Model file for the job. Use its own axes, mm. A direction names the side the tool comes from. Give positions to 0.01 mm unless a question says otherwise; leave off trailing zeros. Write each loop counter-clockwise with the first axis right and the second up, starting at its lowest first coordinate (ties: lowest second). Pieces come first, ordered by that corner, then holes.
```python
from build123d import *

# Parameters (mm, degrees)
F2_R      = 0.3
F3_DEPTH  = 2
F4_DEPTH  = 25
F5_R      = 0.3
F6_ANGLE  = 90
F6_FACE_R = 0.3
F7_R      = 0.3
F8_DEPTH  = 3


# Not quite as in the source:
# - a feature names something its author has since deleted; it is built from what else it names


with BuildPart() as f1:
    # F0 (on Front) → F1 (revolve)
    with BuildSketch(Plane.XZ):
        with BuildLine():
            Line((0, 3.6), (0, 0))
            Line((0, 0), (1.5, 0))
            Line((1.5, 0), (2, 0))
            Line((2, 0), (2, 1))
            Line((2, 1), (1.5, 1))
            Line((1.5, 1), (1.5, 3.6))
            ThreePointArc((1.5, 3.6), (1.0606601718, 4.6606601718), (0, 5.1))
            Line((0, 5.1), (0, 3.6))
        make_face()
    revolve(axis=Axis((0, 0, 1.8), (0, 0, 1)))

    # F2 (on Top) → F3 (join)
    with BuildSketch(Plane.XY):
        with Locations((-1.27, 0)):
            Circle(F2_R)
        with Locations((1.27, 0)):
            Circle(F2_R)
    extrude(amount=-F3_DEPTH)

    # F2 (on Top) → F4 (cut)
    with BuildSketch(Plane.XY):
        with BuildLine():
            Line((1.65, 1.1302654555), (1.65, 0))
            Line((1.65, 0), (1.65, -1.1302654555))
            ThreePointArc((1.65, -1.1302654555), (1.9104973175, -0.5916079783), (2, 0))
            ThreePointArc((2, 0), (1.9104973175, 0.5916079783), (1.65, 1.1302654555))
        make_face()
    extrude(amount=F4_DEPTH, mode=Mode.SUBTRACT)

    # F5 (on face) → F6 (revolve)
    with BuildSketch(Plane(origin=(0, 0, -2), x_dir=(1, 0, 0), z_dir=(0, 0, -1))):
        with Locations((-1.27, 0)):
            Circle(F5_R)
        with Locations((1.27, 0)):
            Circle(F5_R)
    revolve(axis=Axis((0.0564431539, 1.5424509184, -2), (1, 0, 0)), revolution_arc=F6_ANGLE)

    # F6_face (on face) + F7 (on face) → F8 (join)
    with BuildSketch(Plane(origin=(1.27, 1.5424509184, -3.5424509184), x_dir=(-1, 0, 0), z_dir=(0, 1, 0))):
        with Locations((2.54, 0)):
            Circle(F6_FACE_R)
    with BuildSketch(Plane(origin=(0, 1.5424509184, 0), x_dir=(-1, 0, 0), z_dir=(0, 1, 0))):
        with Locations((-1.27, -3.5424509184)):
            Circle(F7_R)
    extrude(amount=F8_DEPTH)


solid = f1.part
```
1. Slice it at B-B, the plane z = -1.5. Write the cut outline in (x, y).
Calculated:
outline: circle Ø0.6 at (-1.27, 0); circle Ø0.6 at (1.27, 0)
2. Pull direction Z, two halves, no side cores. Call faces 3 (the cylindrical face through (-2, 0.07, 0.51)), 4 (the flat face through (0, 0, 0)): +Z half, -Z half, draft (parallel to the pull), parting line (faces both ways), or undercut.
Calculated:
face 3: draft
face 4: undercut
3. Slice it at C-C, the plane y = -0.75. Write the cut outline in (x, z), and give its area (3 significant figures).
Calculated:
outline: (-1.85, 0) - (1.65, 0) - (1.65, 1) - (1.3, 1) - (1.3, 3.6) arc R1.3 ccw to (-1.3, 3.6) - (-1.3, 1) - (-1.85, 1) - close
area: 12.9 mm2
4. Pin check, flat tips, straight feed: P1, Ø2, axis at x = 1.5, y = 3, coming from the -Z side; P2, Ø1.8, axis at x = -0.5, y = 1, coming from the +Z side; P3, Ø2, axis at x = -1.5, z = 2.5, coming from the +Y side; P4, Ø2, axis at y = 0.5, z = 4, coming from the +X side. Stop position of each tip, or through.
Calculated:
P1: stops at z = -3.84
P2: stops at z = 5.08
P3: stops at y = 1.41
P4: stops at x = 1.5
5. Probe probe 1 along Z at (x, y) = (1.25, 2.25); probe 2 along Z at (x, y) = (-1.65, -0.5); probe 3 along Z at (x, y) = (1.4, 1.25). List the from-to ranges inside material, lowest first.
Calculated:
probe 1: z = -3.84 to -3.24
probe 2: z = 0 to 1
probe 3: z = -3.79 to -3.24, 0 to 1
6. Slice it at D-D, the plane z = 2. Write the cut outline in (x, y).
Calculated:
outline: circle Ø3 at (0, 0)
7. Which spindle directions (+Z, -Z, +X, -X, +Y, -Y) get a long thin tool onto all of the face, cutting with end or side? Do faces 1 (the cylindrical face through (-1.5, 0.07, 2.32)), 2 (the flat face through (1.65, 0, 0.5)). Say none if no direction does.
Calculated:
face 1: +Z
face 2: +Z, -Z, +X, +Y, -Y
8. Slice it at A-A, the plane x = 0. Write the cut outline in (y, z), and give its area (3 significant figures).
Calculated:
outline: (-2, 0) - (2, 0) - (2, 1) - (1.5, 1) - (1.5, 3.6) arc R1.5 ccw to (-1.5, 3.6) - (-1.5, 1) - (-2, 1) - close
area: 15.3 mm2
